Geometry: final body of the model. Coordinates: model frame, mm. Round coordinates to 2 decimals unless told otherwise and drop trailing zeros. Write each loop counter-clockwise with the first axis right and the second up, starting at its lowest first coordinate (ties: lowest second). Pieces come first, ordered by that corner, then holes. Notation, with made-up numbers: M 57,-11 L 82,-11 A19 ccw 82,5 Z; hole C 55.5,-23 d2. An arc over 180 degrees is marked long. Answer as CSV lines item,"result". Start each with the question number.
Q1. Ray query, probe 1 along Y at (x, z) = (-10, 0.3); probe 2 along X at (y, z) = (22, -1.25); probe 3 along X at (y, z) = (67.5, 1.2). Return the intervals inside material, ascending.
Q2. Section query B-B on x = -24. Output: boundary loops of the cut face in (y, z).
Q3. First-contact query: pin 1 (1.5 mm diameter, centred on y = 22.5, z = 0.5, fed in from +X). Flat tip, straight axial feed; report the tip coordinate or a pass-through.
Q4. Section query A-A on y = -21. Output: boundary loops of the cut face in (x, z), and give its area (3 significant figures).
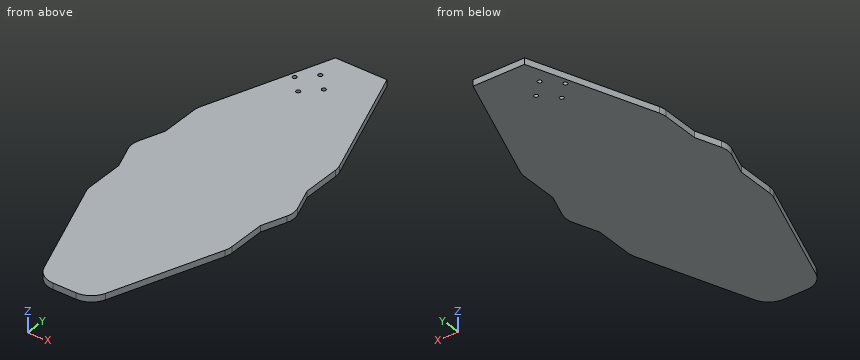
```python
from build123d import *

# Parameters (mm, degrees)
F1_DEPTH = 1.5
F2_R     = 10
F4_D     = 2


with BuildPart() as f1:
    # F0 (on Top) → F1 (new body, symmetric)
    with BuildSketch(Plane.XY):
        Polygon((-34.338214056, 35), (-34.338214056, 15), (-39.79776757, 0), (-34.338214056, -15), (-34.338214056, -35), (-12.5, -95), (0, -95), (12.5, -95), (34.338214056, -35), (34.338214056, -15), (39.79776757, 0), (34.338214056, 15), (34.338214056, 35), (12.5, 95), (0, 95), (-12.5, 95), align=None)
    extrude(amount=F1_DEPTH, both=True)

    # F2
    f2_edges = [f1.edges().sort_by_distance(p)[0] for p in [
        (-34.338214, 35, 0),
        (-39.797768, 0, 0),
        (34.338214, 35, 0),
        (39.797768, 0, 0),
        (-34.338214, -35, 0),
        (34.338214, -35, 0),
        (12.5, -95, 0),
        (-12.5, -95, 0),
    ]]
    fillet(f2_edges, radius=F2_R)

    # F4 (through all)
    with Locations(Plane.XY.offset(1.5)):
        with Locations((-17.0710678119, 74.9289321881), (-10, 82), (-10, 67.8578643763), (-2.9289321881, 74.9289321881)):
            Hole(F4_D / 2)


solid = f1.part
```
Entries:
1,probe 1,"y = -93.93 to 66.86, 68.86 to 81, 83 to 95"
1,probe 2,"x = -34.34 to 34.34"
1,probe 3,"x = -22.51 to -10.93, -9.07 to 22.51"
2,outline,"M -63.4,-1.5 L 63.4,-1.5 L 63.4,1.5 L -63.4,1.5 Z"
3,pin 1,"stops at x = 34.34"
4,outline,"M -34.34,-1.5 L 34.34,-1.5 L 34.34,1.5 L -34.34,1.5 Z"
4,area,"206 mm^2"
